```python
from build123d import *

# Parameters (mm, degrees)
EXTRUDE_1_DEPTH = 4


with BuildPart() as part:
    # Эскиз1 → Бобышка-Вытянуть1 (new body)
    with BuildSketch(Plane.XY):
        Polygon((4.618802154, 0), (2.309401077, 4), (-2.309401077, 4), (-4.618802154, 0), (-2.309401077, -4), (2.309401077, -4), align=None)
    extrude(amount=EXTRUDE_1_DEPTH)

    # Эскиз2 → Вырез-Повернуть2 (revolve, cut)
    with BuildSketch(Plane(origin=(0, 0, 0), x_dir=(1, 0, 0), z_dir=(0, 1, 0))):
        Polygon((-4.018802154, 0), (-4.018802154, 0.812802913), (-5.016585269, 0.812802913), (-5.016585269, -4.215003636), (-4.018802154, -4.215003636), (-4.018802154, -4), (-4.618802154, -3.653589838), (-4.618802154, -0.346410162), align=None)
    revolve(axis=Axis((0, 0, 0), (0, 0, 1)), mode=Mode.SUBTRACT)

    # Эскиз3 → Отверстие обработанное метчиком M51 (revolve, cut)
    with BuildSketch(Plane.YZ):
        Polygon((0, 0), (0, 4), (2.65, 4), (2.1, 3.614885854), (2.1, 0.385114146), (2.65, 0), align=None)
    revolve(axis=Axis((0, 0, -6.35), (0, 0, 1)), mode=Mode.SUBTRACT)


solid = part.part
```
Geometry check sheet. Reference: the model listing, model coordinates, mm. Coordinates: 2 decimals unless noted, no trailing zeros. Order: outer loops, then holes, each group sorted by start corner. A loop starts at its lowest first (then second) coordinate and runs counter-clockwise, first axis right, second up.
Item 1: Section check B-B (z = 1.05). Enter the section's corners in (x, y), plus the area to 3 significant figures.
Item 2: Section check A-A (x = 0). Enter the section's corners in (y, z).
Item 3: Mould release check, pull along Y, two halves, no side actions. Record for faces 1 (the flat face through (3.48, 1.97, 1.97)), 2 (the conical face through (2.075, -3.611, 3.916)), 3 (the cylindrical face through (-0.631, 2.003, 1.977)): released by +Y, released by -Y, zero draft, split by the parting line, or undercut.
Item 4: Depth check by flat-ended pin: pin 1 (2.5 mm diameter, centred on x = 0, y = 0, fed in from -Z). Enter the tip coordinate at first touch or a pass-through.
Item 5: Scan lines: line 1 along Y through (x, z) = (0, 0.45); line 2 along X through (y, z) = (-1.5, 2.6); line 3 along Y through (x, z) = (1.75, 3.25). Record each from-to range of solid material in increasing order.
Check sheet entries:
1. outline: (-4.62, 0) - (-2.31, -4) - (2.31, -4) - (4.62, 0) - (2.31, 4) - (-2.31, 4) - close; hole circle Ø4.2 at (0, 0)
1. area: 41.6 mm2
2. outline: (-4, 0) - (-2.65, 0) - (-2.1, 0.39) - (-2.1, 3.61) - (-2.65, 4) - (-4, 4) - close; (2.1, 0.39) - (2.65, 0) - (4, 0) - (4, 4) - (2.65, 4) - (2.1, 3.61) - close
3. face 1: released by +Y
3. face 2: released by -Y
3. face 3: undercut
4. pin 1: passes through
5. line 1: y = -4 to -2.1, 2.1 to 4
5. line 2: x = -3.75 to -1.47, 1.47 to 3.75
5. line 3: y = -4 to -1.16, 1.16 to 4
